```python
from build123d import *

# Parameters (mm, degrees)
SKETCH_1_R          = 7.9
EXTRUDE_1_DEPTH     = 20
SKETCH_6_R          = 10
EXTRUDE_2_DEPTH     = 2.5
SKETCH_7_R          = 3.5
CUT_EXTRUDE_3_DEPTH = 2.5
CHAMFER_1_SIZE      = 1


with BuildPart() as part:
    # 草图1 → 凸台-拉伸1 (new body)
    with BuildSketch(Plane(origin=(0, 0, 0), x_dir=(0, 0, -1), z_dir=(1, 0, 0))):
        Circle(SKETCH_1_R)
    extrude(amount=-EXTRUDE_1_DEPTH)

    # 草图6 → 凸台-拉伸2 (add)
    with BuildSketch(Plane(origin=(0, 0, 0), x_dir=(0, 0, -1), z_dir=(1, 0, 0))):
        Circle(SKETCH_6_R)
    extrude(amount=EXTRUDE_2_DEPTH)

    # 草图7 → 切除-拉伸3 (cut)
    with BuildSketch(Plane(origin=(2.5, 0, 0), x_dir=(0, 0, -1), z_dir=(1, 0, 0))):
        Circle(SKETCH_7_R)
    extrude(amount=-CUT_EXTRUDE_3_DEPTH, mode=Mode.SUBTRACT)

    # 倒角1
    chamfer_1_edges = [part.edges().sort_by_distance(p)[0] for p in [
        (2.5, 0, 10),
    ]]
    chamfer(chamfer_1_edges, length=CHAMFER_1_SIZE)


solid = part.part
```
Design review of the part built by this model. Coordinates are the model's own, in mm. A direction names the side the tool comes from. Give positions to 0.01 mm unless a question says otherwise; leave off trailing zeros. Write each loop counter-clockwise with the first axis right and the second up, starting at its lowest first coordinate (ties: lowest second). Pieces come first, ordered by that corner, then holes.
(1) Add section A-A (y = 0). Give the boundary of the cut face in (x, z).
Checked values:
outline: (-20, -7.9) - (0, -7.9) - (0, -10) - (1.5, -10) - (2.5, -9) - (2.5, -3.5) - (0, -3.5) - (0, 3.5) - (2.5, 3.5) - (2.5, 9) - (1.5, 10) - (0, 10) - (0, 7.9) - (-20, 7.9) - close
(2) Wall thickness on line 1 along Y through (x, z) = (0.95, 0); line 2 along X through (y, z) = (0, 1.5); line 3 along Y through (x, z) = (0.5, -3): over which ranges is each line inside the solid? List them lowest first.
Checked values:
line 1: y = -10 to -3.5, 3.5 to 10
line 2: x = -20 to 0
line 3: y = -9.54 to -1.8, 1.8 to 9.54
(3) Mouldability with a two-part tool opening along Z and no side actions: class faces 1 (the face through (2.5, -4, 0)), 2 (the face through (0.74, -9.76, 2.17)), 3 (the face through (1.268, -1.341, -3.233)) as +Z half, -Z half, draft (parallel to the pull), parting line (faces both ways), or undercut.
Checked values:
face 1: draft
face 2: parting line
face 3: undercut
(4) Add section C-C (x = -4.5). Give the boundary of the cut face in (y, z).
Checked values:
outline: circle Ø15.8 at (0, 0)
(5) Tool access review of faces 4 (the face through (0, 0, 0)), 5 (the face through (-20, 0, 0)), 6 (the face through (0, -4, -7)): name each direction out of +Z, -Z, +X, -X, +Y, -Y from which nothing blocks a thin tool from reaching the whole face with its end or side.
Checked values:
face 4: +X
face 5: +Z, -Z, -X, +Y, -Y
face 6: -X
(6) Clearance check with flat-ended pins moving along their axes: pin 1 Ø12 at (x, y) = (-13.5, -3.5) entering from -Z; pin 2 Ø8 at (x, y) = (-8, -1.5) entering from +Z; pin 3 Ø2 at (y, z) = (1.5, 1.5) entering from +X; pin 4 Ø3 at (y, z) = (-2.5, -1.5) entering from +X. State where each tip first meets the part, or that it passes through.
Checked values:
pin 1: stops at z = -7.9
pin 2: stops at z = 7.9
pin 3: stops at x = 0
pin 4: stops at x = 2.5
